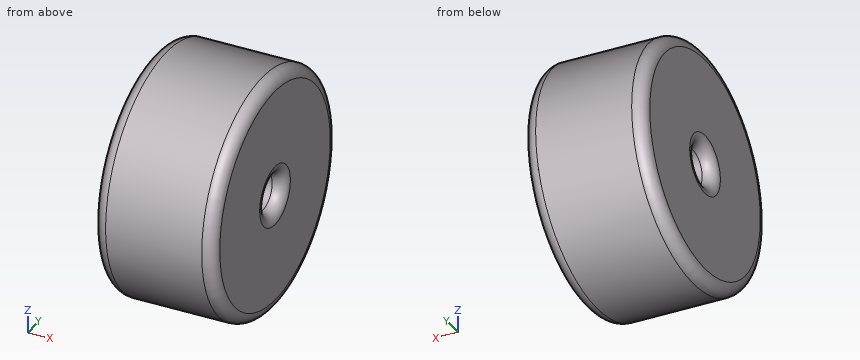
Autodesk Inventor part; units mm, degrees
ref_plane "YZ Plane" through (0, 0, 0) normal (1, 0, 0) x (0, 1, 0)
ref_plane "XZ Plane" through (0, 0, 0) normal (0, 1, 0) x (-1, 0, 0)
ref_plane "XY Plane" through (0, 0, 0) normal (0, 0, 1) x (1, 0, 0)
sketch "草图1" plane through (0, 0, 0) normal (1, 0, 0) x (0, 1, 0)
  circle A0 centre (0, 0) radius 20
  dimension "d0" = 40
extrude "拉伸1" add sketch "草图1" along normal blind 20
sketch "草图2" plane through (20, 0, 0) normal (1, 0, 0) x (0, 0, -1)
  circle A0 centre (0, 0) radius 3
  dimension "d3" = 6
extrude "拉伸2" cut sketch "草图2" against normal through all
fillet "圆角1" radius 2 4 edges at (0, -20, 0) (20, -20, 0) (0, 0, 3) (20, 0, 3)
properties part number "皮带轮"
The listing builds one solid part. Answer for the finished solid, in the listing's coordinates (mm). Coordinates: 2 decimals unless noted, no trailing zeros. Write each loop counter-clockwise with the first axis right and the second up, starting at its lowest first coordinate (ties: lowest second). Pieces come first, ordered by that corner, then holes. Notation, with made-up numbers: M 6.5,1 L 14.5,1 A10 cw 14.5,8 Z; hole C -0.5,22.5 d3. An arc over 180 degrees is marked long. Use a Markdown table: item, result. Add a question column.
1. Straight lines are drawn through the part: line 1 along X through (y, z) = (-1.5, 18); line 2 along Z through (x, y) = (10.25, 1); line 3 along Z through (x, y) = (4.75, 15.5). For each, find the intervals that lie inside material, in ascending order. Write a range as [from, to].
2. Section A-A (y = 0) is taken. Give the vertices of the cut face in (x, z).
3. Section C-C (x = 7.5) is taken. Give the vertices of the cut face in (y, z).
4. Section D-D (x = 18.75) is taken. Give the vertices of the cut face in (y, z).
5. Given P1, Ø3, axis at x = 7.5, z = -6, coming from the +Y side; P2, Ø1.5, axis at x = 16, y = -15.5, coming from the +Z side; P3, Ø1.5, axis at x = 14.5, y = 11, coming from the +Z side; P4, Ø12, axis at y = -7.5, z = 14.5, coming from the -X side, each flat-ended and moving along its own axis, determine where each tip first touches the part or whether it passes through.
Data:
| question | item | result |
|---|---|---|
| 1 | line 1 | x = [0, 20] |
| 1 | line 2 | z = [-19.97, -2.83], [2.83, 19.97] |
| 1 | line 3 | z = [-12.64, 12.64] |
| 2 | outline | M 0,-18 A2 ccw 2,-20 L 18,-20 A2 ccw 20,-18 L 20,-5 A2 ccw 18,-3 L 2,-3 A2 ccw 0,-5 Z; M 0,5 A2 ccw 2,3 L 18,3 A2 ccw 20,5 L 20,18 A2 ccw 18,20 L 2,20 A2 ccw 0,18 Z |
| 3 | outline | C 0,0 d40; hole C 0,0 d6 |
| 4 | outline | C 0,0 d39.71; hole C 0,0 d6.29 |
| 5 | P1 | stops at y = 19.49 |
| 5 | P2 | stops at z = 13.51 |
| 5 | P3 | stops at z = 17.17 |
| 5 | P4 | stops at x = 0 |
